Geometry check sheet. Reference: the model listing, model coordinates, mm. Face numbers are marked on the shaded views. A direction names the side the tool comes from. Round coordinates to 2 decimals unless told otherwise and drop trailing zeros. Write each loop counter-clockwise with the first axis right and the second up, starting at its lowest first coordinate (ties: lowest second). Pieces come first, ordered by that corner, then holes. Notation, with made-up numbers: M 29,12 L 74,12 A34 cw 74,49 Z; hole C -24,89 d1. An arc over 180 degrees is marked long. One line per item, written item: value. Start each with the question number.
1. Depth check by flat-ended pin: P1, Ø2, axis at x = 4, z = 0, coming from the -Y side; P2, Ø5, axis at x = 19.5, y = -3, coming from the +Z side; P3, Ø3, axis at x = 20, y = -2, coming from the -Z side. Enter the tip coordinate at first touch or a pass-through.
2. Section check D-D (x = 11). Record the boundary of the cut face in (y, z).
3. Section check C-C (y = -1.5). Record the boundary of the cut face in (x, z), and give its area (3 significant figures).
4. Access from +Z, -Z, +X, -X, +Y, -Y to the whole of each face (thin tool, end or side, straight path). Record for the marked faces 1, 2, 3 and 4.
5. Section check B-B (z = -1.75). Record the boundary of the cut face in (x, y).
6. Section check A-A (x = 18). Record the boundary of the cut face in (y, z), and give its area (3 significant figures).
7. Scan lines: probe 1 along Z at (x, y) = (13.5, 1); probe 2 along Y at (x, z) = (11, 0.4); probe 3 along X at (y, z) = (1, 2). Record each from-to range of solid material in increasing order. Write a range as [from, to].
from build123d import *

# Parameters (mm, degrees)
F1_DEPTH = 4
F0_R     = 0.5
F2_DEPTH = 1
F3_R     = 2.5
F3_R_2   = 0.5
F4_DEPTH = 2.5


with BuildPart() as f1:
    # F0 (on Top) → F1 (new body, symmetric)
    with BuildSketch(Plane.XY):
        with BuildLine():
            Line((-3.3166247904, -5), (0, -5))
            Line((0, -5), (3.3166247904, -5))
            ThreePointArc((3.3166247904, -5), (6, 0), (3.3166247904, 5))
            Line((3.3166247904, 5), (-3.3166247904, 5))
            ThreePointArc((-3.3166247904, 5), (-6, 0), (-3.3166247904, -5))
        make_face()
        with BuildLine():
            ThreePointArc((0, -3), (-2.1213203436, 2.1213203436), (3, 0))
            ThreePointArc((3, 0), (2.1213203436, -2.1213203436), (0, -3))
        make_face(mode=Mode.SUBTRACT)
    extrude(amount=F1_DEPTH, both=True)

    # F0 (on Top) → F2 (join, symmetric)
    with BuildSketch(Plane.XY):
        with BuildLine():
            ThreePointArc((3.3166247904, 5), (6, 0), (3.3166247904, -5))
            Line((3.3166247904, -5), (6.6147298804, -5))
            Line((6.6147298804, -5), (25, -2))
            ThreePointArc((25, -2), (26.9998884615, 0.0211220617), (24.9577582326, 1.9995538585))
            Line((24.9577582326, 1.9995538585), (6.2387437176, 5))
            Line((6.2387437176, 5), (3.3166247904, 5))
        make_face()
        with Locations((11, 0)):
            Circle(F0_R, mode=Mode.SUBTRACT)
        with Locations((14.5, 0)):
            Circle(F0_R, mode=Mode.SUBTRACT)
        with Locations((18, 0)):
            Circle(F0_R, mode=Mode.SUBTRACT)
        with Locations((21.5, 0)):
            Circle(F0_R, mode=Mode.SUBTRACT)
        with Locations((25, 0)):
            Circle(F0_R, mode=Mode.SUBTRACT)
    extrude(amount=F2_DEPTH, both=True)

    # F3 (on face) → F4 (join)
    with BuildSketch(Plane.XZ.offset(5)):
        Circle(F3_R)
        Circle(F3_R_2, mode=Mode.SUBTRACT)
    extrude(amount=F4_DEPTH)


solid = f1.part
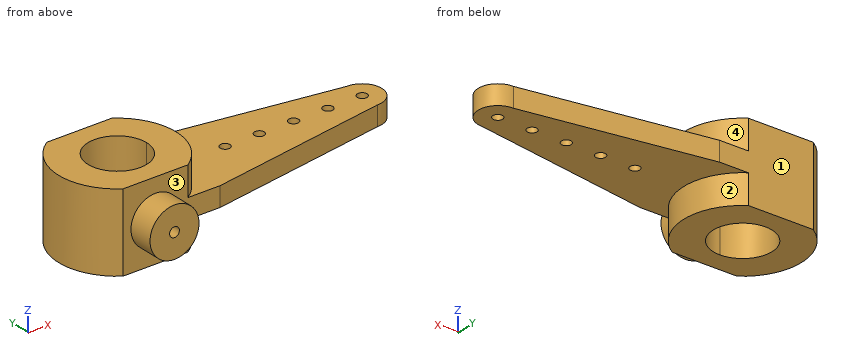
Result sheet:
1. P1: stops at y = -5
1. P2: stops at z = 1
1. P3: stops at z = -1
2. outline: M -4.28,-1 L -0.5,-1 L -0.5,1 L -4.28,1 Z; M 0.5,-1 L 4.24,-1 L 4.24,1 L 0.5,1 Z
3. outline: M -5.81,-4 L -2.6,-4 L -2.6,4 L -5.81,4 Z; M 2.6,-4 L 5.81,-4 L 5.81,-1 L 26.32,-1 L 26.32,1 L 5.81,1 L 5.81,4 L 2.6,4 Z
3. area: 92.4 mm2
4. face 1: +Z, -Z, +X, -X, +Y
4. face 2: -Z, +X
4. face 3: -Y
4. face 4: +Z, +X
5. outline: M -3.32,-5 L -1.79,-5 L -1.79,-7.5 L 1.79,-7.5 L 1.79,-5 L 3.32,-5 A6 ccw 3.32,5 L -3.32,5 A6 ccw Z; hole C 0,0 d6
6. outline: M -3.14,-1 L -0.5,-1 L -0.5,1 L -3.14,1 Z; M 0.5,-1 L 3.11,-1 L 3.11,1 L 0.5,1 Z
6. area: 10.5 mm2
7. probe 1: z = [-1, 1]
7. probe 2: y = [-4.28, -0.5], [0.5, 4.24]
7. probe 3: x = [-5.92, -2.83], [2.83, 5.92]
